The listing builds one solid part. Answer for the finished solid, in the listing's coordinates (mm). A direction names the side the tool comes from. Round coordinates to 2 decimals unless told otherwise and drop trailing zeros. Write each loop counter-clockwise with the first axis right and the second up, starting at its lowest first coordinate (ties: lowest second). Pieces come first, ordered by that corner, then holes. Notation, with made-up numbers: M 7.25,-10.75 L 29.25,-10.75 A30 cw 29.25,15.25 Z; hole C -3,-27 d11. An arc over 180 degrees is marked long. One line per item, written item: value. Start each with the question number.
(1) Section A-A (x = 0.75) is taken. Determine the outline of the cut face in (y, z).
(2) Section B-B (x = 4.75) is taken. Determine the outline of the cut face in (y, z).
(3) For a pull along Y with two mould halves and no side action, classify faces 1 (the flat face through (-1.5, 0.4, 0)), 2 (the cylindrical face through (5.41, -1.5, -0.07)), 3 (the flat face through (10, 0, 0)) as released by +Y, released by -Y, zero draft, split by the parting line, or undercut.
(4) Consider probe 1 along Z at (x, y) = (6.25, 0); probe 2 along X at (y, z) = (-2.3, -1.2). Determine where each line is inside the solid, lowest interval first.
(5) Given P1, Ø1, axis at x = -1.5, z = 0.5, coming from the +Y side; P2, Ø1, axis at x = -1.5, z = -0.5, coming from the -Y side; P3, Ø1, axis at y = -0.5, z = -2, coming from the +X side, each flat-ended and moving along its own axis, determine where each tip first touches the part or whether it passes through.
(6) For faces 4 (the flat face through (-1.5, -0.4, 0)), 5 (the cylindrical face through (-0.159, -0.596, 2.685)), 6 (the cylindrical face through (0.465, 1.244, 0.516)), determine the directions among +Z, -Z, +X, -X, +Y, -Y from which every point of the face is accessible in a straight line to the end or side of a thin tool.
Autodesk Inventor part; units mm, degrees
ref_plane "IDS_WORKPLANE{1}" through (-2.1389, 0, 0) normal (1, 0, 0) x (0, 0, -1)
ref_plane "Work Plane2" through (8.25, 0, 0) normal (0, 0, -1) x (1, 0, 0)
ref_plane "YZ Plane" through (0, 0, 0) normal (1, 0, 0) x (0, 1, 0)
sketch "Skizze1" plane through (0, 0, 0) normal (0, 0, 1) x (1, 0, 0)
  line L0 (-2.1389, 0) -> (10, 0)
  line L1 (10, 0) -> (10, 1.5)
  line L2 (10, 1.5) -> (1.25, 1.5)
  line L3 (1.25, 1.5) -> (0.9433, 1.3468)
  line L4 (0.9433, 1.3468) -> (0, 1.3467)
  line L5 (0, 1.3467) -> (0, 2.75)
  line L6 (-6.0203, 0) -> (20.8022, 0)
  line L7 (0, -0.5507) -> (0, 3.3039)
  line L8 (0, 2.75) -> (-1.94, 2.7497)
  arc A0 (-1.94, 2.7497) -> (-2.1389, 0) centre (16.9704, 0) ccw
  dimension "d0" = 10
  dimension "d1" = 8.75
  dimension "d2" = 0.3067
  dimension "d3" = 2.1389
  dimension "d4" = 3
  dimension "d5" = 2.6935
  dimension "d9" = 5.5
  dimension "d10" = 0.01
  dimension "d15" = 19.1093
revolve "Körper" add sketch "Skizze1" angle 360 about axis through (-2.1389, 0, 0) along (1, 0, 0)
fillet "Rundung1" radius 1.8 1 edges at (-1.94, -2.7497, 0)
ref_plane "IDS_WORKPLANE{1}" through (-2.1389, 0, 0) normal (1, 0, 0) x (0, 0, -1)
sketch "Skizze2" plane through (-2.1389, 0, 0) normal (1, 0, 0) x (0, 0, -1)
  line L0 (0, -3.85) -> (0, 3.85)
  line L1 (3.85, 0) -> (-3.85, 0)
  line L2 (-2.75, 0.4) -> (2.75, 0.4)
  line L3 (2.75, 0.4) -> (2.75, -0.4)
  line L4 (2.75, -0.4) -> (-2.75, -0.4)
  line L5 (-2.75, -0.4) -> (-2.75, 0.4)
  line L6 (0, 0.4) -> (0, -0.4) construction
  line L7 (-2.75, 0) -> (2.75, 0) construction
  circle A0 centre (0, 0) radius 2.75
  dimension "d17" = 0.8
extrude "Loch" cut sketch "Skizze2" along normal blind 1.2 contours L4 A0 L1 L0 | L0 L1 A0 L4 | L4 L5 A0 | A0 L3 L4 | L1 A0 L2 L0 | L0 L2 A0 L1 | L5 L2 A0 | A0 L2 L3
thread "Gewinde"
chamfer "Fase1" distance 0.3067 distance2 0.3068 1 edges at (10, -1.5, 0) measured on face at (10, 0.417, 0.2189)
ref_plane "Work Plane2" through (8.25, 0, 0) normal (0, 0, -1) x (1, 0, 0)
equation "\"d0\" = NLG"
equation "\"d1\" = GEL"
equation "\"d2\" = GAL"
equation "\"d3\" = KOH"
equation "\"d4\" = GD"
equation "\"d5\" = BDM"
equation "\"d9\" = KOD"
equation "\"d10\" = KEWI"
equation "\"d17\" = SBR"
equation "\"d18\" = STI"
equation "\"d20\" = RR"
equation "\"d11\" = GEL"
equation "\"d13\" = -0.5 * SPD + 0.5 * GD"
equation "\"GD\" = NND"
equation "\"NLG\" = 10"
equation "\"GEL\" = 8.75"
equation "\"KOD\" = 5.5"
equation "\"KOH\" = 2.13889"
equation "\"GAL\" = 0.61345 * PTC"
equation "\"SPD\" = NND - 1.2269 * PTC"
equation "\"BDM\" = 2.6935"
equation "\"GUL\" = 0.61345 * PTC"
equation "\"RR\" = 1.8"
equation "\"SBR\" = 0.8"
equation "\"STI\" = 1.2"
equation "\"KEWI\" = 0.01deg"
equation "\"KR\" = 3.3"
equation "\"d16\" = -KOH"
equation "\"PTC\" = 0.5"
equation "\"THREADDIA\" = 3"
equation "\"TOA\" = 30deg"
equation "\"NND\" = 3"
equation "\"ORI\" = 1.8"
equation "\"GD1\" = THREADDIA - 1.2269 * PTC"
properties part number "CNS 9671 - M3 x 10" material "Steel, Mild"
Recorded:
1. outline: C 0,0 d2.69
2. outline: C 0,0 d3
3. face 1: undercut
3. face 2: split by the parting line
3. face 3: zero draft
4. probe 1: z = -1.5 to 1.5
4. probe 2: x = -1.05 to 0
5. P1: stops at y = 2.58
5. P2: stops at y = -2.58
5. P3: stops at x = 0
6. face 4: +Z, -Z, -X
6. face 5: +X, -X
6. face 6: none
